Geometry: see drawing. Coordinates: mm, zero at the bounding-box minimum. Give positions to 0.01 mm unless a question says otherwise; leave off trailing zeros. Write each loop counter-clockwise with the first axis right and the second up, starting at its lowest first coordinate (ties: lowest second). Pieces come first, ordered by that corner, then holes. Notation, with made-up numbers: (75, -22.5) -> (85, -22.5) arc R34 cw to (85, 7.5) -> close; hole circle Ø8 at (36, 51.5). An arc over 180 degrees is marked (long way). Answer as a JSON object with one key per item and string values. Group by question number.
Item 1: Section query A-A on z = 205. Return the cut outline in (x, y).
Item 2: First-contact query: pin 1 Ø3 at (y, z) = (3.5, 30.5) entering from -X; pin 2 Ø3 at (y, z) = (1.5, 50.5) entering from +X. Flat tips, straight axial feed; report the tip coordinate or a pass-through.
Item 3: Section query B-B on x = 47. Return the cut outline in (y, z).
Item 4: Ray query, probe 1 along Z at (x, y) = (56.5, 1.95); probe 2 along X at (y, z) = (4.45, 41). Return the intervals inside material, ascending. Write a range as from..to.
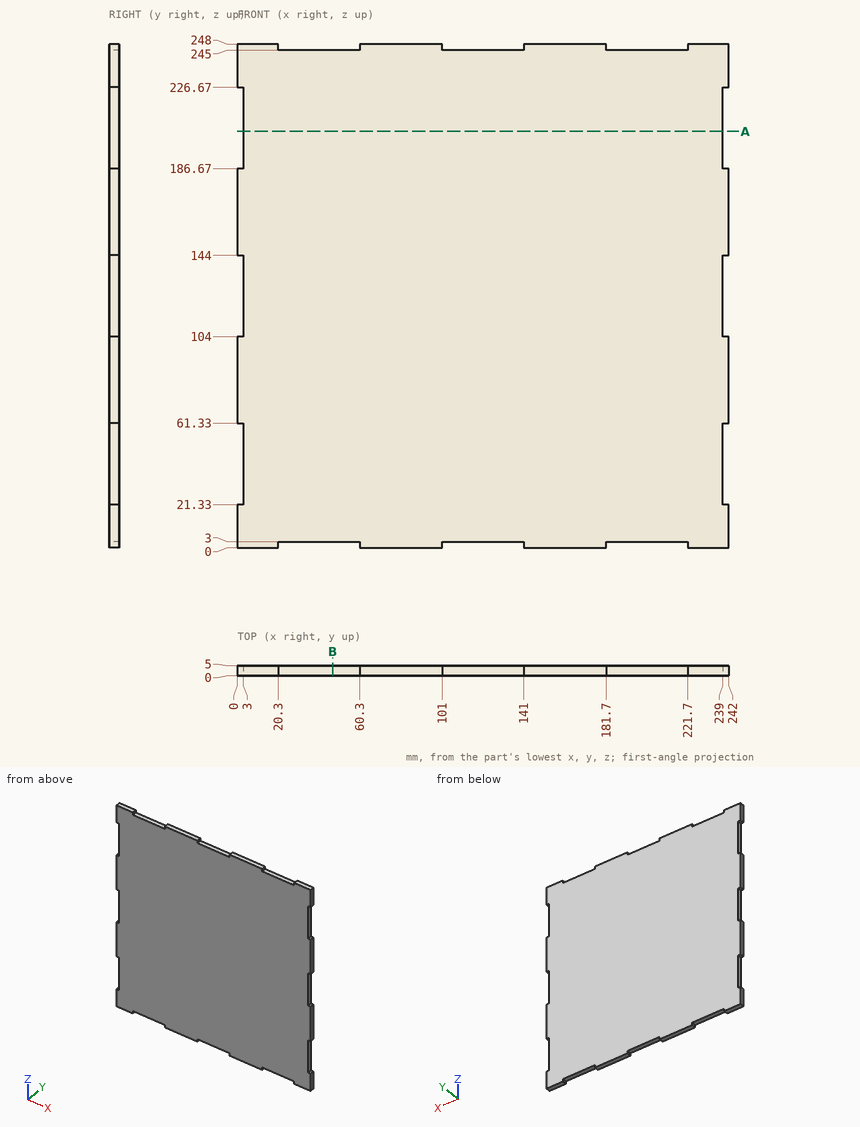
Worked answers:
{
 "1": {"outline": "(3, 0) -> (239, 0) -> (239, 5) -> (3, 5) -> close"},
 "2": {"pin 1": "x = 3", "pin 2": "x = 239"},
 "3": {"outline": "(0, 3) -> (5, 3) -> (5, 245) -> (0, 245) -> close"},
 "4": {"probe 1": "3..245", "probe 2": "3..239"}
}
